Verification items for the finished model (mm, model axes). A direction names the side the tool comes from. Give positions to 0.01 mm unless a question says otherwise; leave off trailing zeros. Loops run counter-clockwise (first coordinate to the right, second up) from the corner with the lowest first, then second, coordinate; pieces in that order, holes last. Notation, with made-up numbers: M 16,-15 L 52,-15 A19 cw 52,2 Z; hole C 70.25,79 d4. An arc over 180 degrees is marked long. Use a Markdown table: item, result.
from build123d import *

# Parameters (mm, degrees)
SKETCH144_W             = 42.5
SKETCH144_H             = 29
SKETCH144_R             = 10
PAD034_DEPTH            = 3
PAD036_DEPTH            = 2.4
FILLET021_R             = 5
CHAMFER004_SIZE         = 1
BODY013_PLACEMENT_ANGLE = 20


with BuildPart() as part:
    # Sketch144 → Pad034 (new body)
    with BuildSketch(Plane.XY):
        Rectangle(SKETCH144_W, SKETCH144_H)
        Circle(SKETCH144_R, mode=Mode.SUBTRACT)
    extrude(amount=PAD034_DEPTH)

    # Sketch146 (on Face3 of Pad034) → Pad036 (join, symmetric)
    with BuildSketch(Plane(origin=(0, 0, 0), x_dir=(-1, 0, 0), z_dir=(0, 1, 0))):
        Polygon((16.25, 3), (18.25, 3), (18.25, 7), (19.25, 7), (19.25, 8.5), (18.25, 10), (16.25, 10), align=None)
    pad036 = extrude(amount=PAD036_DEPTH, both=True)

    # Mirrored010: Pad036 across Sketch146 V_Axis
    add(pad036.mirror(Plane(origin=(0, 0, 0), x_dir=(0, 1, 0), z_dir=(-1, 0, 0))))

    # Fillet021
    fillet021_edges = [part.edges().sort_by_distance(p)[0] for p in [
        (21.25, 14.5, 1.5),
        (-21.25, 14.5, 1.5),
        (-21.25, -14.5, 1.5),
        (21.25, -14.5, 1.5),
    ]]
    fillet(fillet021_edges, radius=FILLET021_R)

    # Chamfer004
    chamfer004_edges = [part.edges().sort_by_distance(p)[0] for p in [
        (0, 14.5, 0),
    ]]
    chamfer(chamfer004_edges, length=CHAMFER004_SIZE)


with BuildPart() as part_1:
    # Body013 placement: moved
    add(part.part.moved(Location((-357.518507, 122.995147, 204.709932))).rotate(Axis((-357.518507, 122.995147, 204.709932), (1, 0, 0)), BODY013_PLACEMENT_ANGLE))


solid = part_1.part
(1) Material ranges on line 1 (X direction, y = 119.75, z = 207.25); line 2 (X direction, y = 115.5, z = 204.5); line 3 (Z direction, x = -368, y = 134), recorded low to high.
Results below:
| item | result |
|---|---|
| line 1 | -375.77 to -373.77, -341.27 to -339.27 |
| line 2 | -378.77 to -364.55, -350.49 to -336.27 |
| line 3 | 208.72 to 211.91 |
(2) Cross-section at A-A on x = -358.5. Record the cut outline in (y, z).
Results below:
| item | result |
|---|---|
| outline | M 108.34,202.57 L 109.03,200.69 L 110.31,200.09 L 113.64,201.31 L 112.62,204.13 Z; M 131.32,210.93 L 132.35,208.11 L 135.68,209.33 L 136.28,210.61 L 135.59,212.49 Z |
(3) Gauge pin test, flat ends, axial feed: P1, Ø6, axis at y = 121, z = 210.5, coming from the -X side; P2, Ø6, axis at x = -354, z = 204.5, coming from the +Y side; P3, Ø3, axis at y = 117.5, z = 202, coming from the -X side. Record the tip position at first contact, or that the pin passes through.
Results below:
| item | result |
|---|---|
| P1 | x = -376.77 |
| P2 | y = 115.22 |
| P3 | x = -378.6 |
(4) Cross-section at C-C on x = -351.5. Record the cut outline in (y, z), then the cut area to 3 significant figures.
Results below:
| item | result |
|---|---|
| outline | M 108.34,202.57 L 109.03,200.69 L 110.31,200.09 L 115.49,201.98 L 114.46,204.8 Z; M 129.47,210.26 L 130.5,207.44 L 135.68,209.33 L 136.28,210.61 L 135.59,212.49 Z |
| area | 38.1 mm^2 |
(5) Set-up check for faces 5 (the flat face through (-376.769, 120, 212)), 6 (the cylindrical face through (-367.51, 122.9, 206.25)), 7 (the flat face through (-340.123, 123.011, 211.685)): record each of +Z, -Z, +X, -X, +Y, -Y from which the full face is reachable in a straight line by a thin tool's end or side.
Results below:
| item | result |
|---|---|
| face 5 | +Z, -X, -Y |
| face 6 | none |
| face 7 | +Z, +X, -X |
(6) Draft check along Y on faces 1 (the flat face through (-357.291, 109.659, 200.396)), 2 (the flat face through (-362.302, 131.63, 207.853)), 3 (the flat face through (-376.26, 120.63, 211.3)), 4 (the flat face through (-338.269, 120, 212)). Enter one of: +Y half, -Y half, draft (parallel to the pull), parting line (faces both ways), or undercut.
Results below:
| item | result |
|---|---|
| face 1 | -Y half |
| face 2 | +Y half |
| face 3 | undercut |
| face 4 | draft |
(7) Cross-section at B-B on x = -372. Record the cut outline in (y, z), then the cut area to 3 significant figures.
Results below:
| item | result |
|---|---|
| outline | M 108.34,202.57 L 109.03,200.69 L 110.31,200.09 L 135.68,209.33 L 136.28,210.61 L 135.59,212.49 Z |
| area | 86.0 mm^2 |
